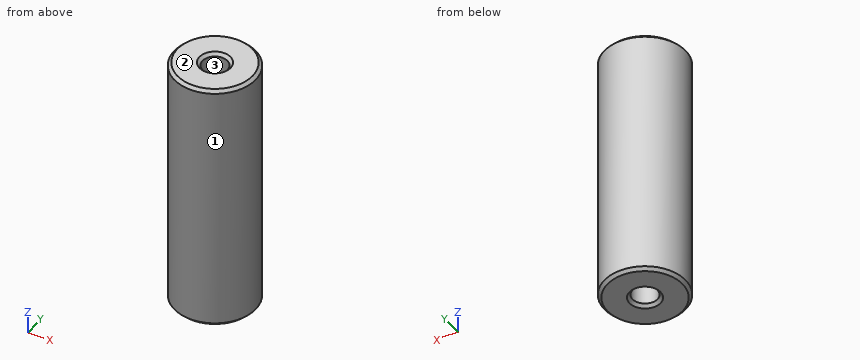
Autodesk Inventor part; units mm, degrees
ref_plane "YZ Plane" through (0, 0, 0) normal (1, 0, 0) x (0, 1, 0)
ref_plane "XZ Plane" through (0, 0, 0) normal (0, 1, 0) x (-1, 0, 0)
ref_plane "XY Plane" through (0, 0, 0) normal (0, 0, 1) x (1, 0, 0)
sketch "スケッチ1" plane through (0, 0, 0) normal (0, 0, 1) x (1, 0, 0)
  circle A0 centre (0, 0) radius 4
  dimension "d0" = 8
extrude "押し出し1" add sketch "スケッチ1" along normal mid plane 25
sketch "スケッチ2" plane through (0, 0, -12.5) normal (0, 0, -1) x (-1, 0, 0)
  point P0 (0, 0)
hole "穴1" at (0, 0, -12.5) direction (0, 0, 1) diameter 2.459 end through all
thread "ねじ1"
chamfer "面取り1" distance 0.3 angle 45 4 edges at (0, -1.2295, -12.5) (-4, 0, -12.5) (0, -1.2295, 12.5) (-4, 0, 12.5)
properties part number "ラックギア側ベアリング軸" material "アルミニウム 2014-T4"
Here's how the part is built. I have some questions about the finished solid (model axes, mm). Face numbers are marked on the shaded views. Round coordinates to 2 decimals unless told otherwise and drop trailing zeros. Loops run counter-clockwise (first coordinate to the right, second up) from the corner with the lowest first, then second, coordinate; pieces in that order, holes last. Notation, with made-up numbers: (27.25, 39.25) -> (36.25, 39.25) arc R18 cw to (36.25, 53.25) -> close; hole circle Ø3 at (8.25, 43.5). An arc over 180 degrees is marked (long way). Answer as CSV lines item,"result".
1. If we section it at C-C on z = -9.5: Please give me the cut outline in (x, y).
Final values:
outline,"circle Ø8 at (0, 0); hole circle Ø2.46 at (0, 0)"
2. For pin 1 (4 mm diameter, centred on x = 3, z = 3, fed in from -Y); pin 2 (1.5 mm diameter, centred on y = 2, z = -6.5, fed in from -X); pin 3 (3 mm diameter, centred on x = 0, y = 0, fed in from +Z), each with a flat end and sliding along its axis, tell me the tip position at first contact or that it passes through.
Final values:
pin 1,"stops at y = -3.87"
pin 2,"stops at x = -3.8"
pin 3,"stops at z = 12.47"
3. If we section it at A-A on y = 0: Please give me the cut outline in (x, z).
Final values:
outline,"(-4, -12.2) -> (-3.7, -12.5) -> (-1.53, -12.5) -> (-1.23, -12.2) -> (-1.23, 12.2) -> (-1.53, 12.5) -> (-3.7, 12.5) -> (-4, 12.2) -> close; (1.23, -12.2) -> (1.53, -12.5) -> (3.7, -12.5) -> (4, -12.2) -> (4, 12.2) -> (3.7, 12.5) -> (1.53, 12.5) -> (1.23, 12.2) -> close"
4. Thinking about a two-plate mould opening in X: for the marked faces 1, 2 and 3, which applies, released by +X, released by -X, zero draft, split by the parting line, or undercut?
Final values:
face 1,"split by the parting line"
face 2,"zero draft"
face 3,"undercut"
5. If I drill on L1, parallel to Y at x = 0, z = 4.75; L2, parallel to Y at x = -0.5, z = 6.5, over which ranges is the centre line in solid material (lowest first)?
Final values:
L1,"y = -4 to -1.23, 1.23 to 4"
L2,"y = -3.97 to -1.12, 1.12 to 3.97"
